from build123d import *

# Parameters (mm, degrees)
F1_DEPTH = 31.75
F2_DEPTH = 92.075
F0_R     = 15.875
F3_DEPTH = 53.975
F4_DEPTH = 73.025
F5_SCALE = 0.5


with BuildPart() as f1:
    # F0 (on Top) → F1 (new body)
    with BuildSketch(Plane.XY):
        Polygon((69.8498128911, -44.4499999985), (69.85, -76.2), (127, -76.2), (127, -25.4), (111.125, -25.4), (111.1241018772, 25.4), (126.9991018772, 25.4), (126.9991018772, 76.2), (69.8491018772, 76.2), (69.8492889861, 44.45), align=None)
    extrude(amount=F1_DEPTH)

    # F0 (on Top) → F2, piece 2 (join)
    with BuildSketch(Plane.XY):
        Polygon((38.1, 76.2), (38.1, 44.4498128953), (69.8492889861, 44.45), (69.8491018772, 76.2), align=None)
        Polygon((38.1, -44.4501871063), (38.1, -76.2), (69.85, -76.2), (69.8498128911, -44.4499999985), align=None)
    extrude(amount=F2_DEPTH)



with BuildPart() as f1b:
    # F0 (on Top) → F1, piece 2 (new body)
    with BuildSketch(Plane.XY):
        Polygon((-111.125, -25.4), (-127, -25.4), (-127, -76.2), (-69.85, -76.2), (-69.8501871089, -44.45), (-69.8507110139, 44.45), (-69.8508981228, 76.2), (-127.0008981228, 76.2), (-127.0008981228, 25.4), (-111.125, 25.4), align=None)
    extrude(amount=F1_DEPTH)

    # F0 (on Top) → F2 (join)
    with BuildSketch(Plane.XY):
        Polygon((-69.8508981228, 76.2), (-69.8507110139, 44.45), (-38.1, 44.45), (-38.1, 76.2), align=None)
        Polygon((-69.8501871089, -44.45), (-69.85, -76.2), (-38.1, -76.2), (-38.1, -44.45), align=None)
    extrude(amount=F2_DEPTH)


with BuildPart() as f1_1:
    add(f1.part)

    add(f1b.part)  # F3 merges F1b
    # F0 (on Top) → F3 (join)
    with BuildSketch(Plane.XY):
        Polygon((-38.1, -44.45), (-38.1, -76.2), (0, -76.2), (38.1, -76.2), (38.1, -44.4501871063), (38.1, 44.4498128953), (38.1, 76.2), (-38.1, 76.2), (-38.1, 44.45), align=None)
        Circle(F0_R, mode=Mode.SUBTRACT)
    extrude(amount=F3_DEPTH)

    # F0 (on Top) → F4 (join)
    with BuildSketch(Plane.XY):
        Polygon((38.1, 44.4498128953), (38.1, -44.4501871063), (69.8498128911, -44.4499999985), (69.8492889861, 44.45), align=None)
        Polygon((-69.8507110139, 44.45), (-69.8501871089, -44.45), (-38.1, -44.45), (-38.1, 44.45), align=None)
    extrude(amount=F4_DEPTH)


with BuildPart() as f1_2:
    # F5: moved
    add(f1_1.part.scale(F5_SCALE))


solid = f1_2.part
Design review of the part built by this model. Coordinates are the model's own, in mm. A direction names the side the tool comes from. Coordinates: 2 decimals unless noted, no trailing zeros. Order: outer loops, then holes, each group sorted by start corner. A loop starts at its lowest first (then second) coordinate and runs counter-clockwise, first axis right, second up.
Item 1: Take a section at A-A, the plane z = 29. Write out the cut boundary in (x, y) (3 decimals), then the cut area to 3 significant figures.
Item 2: For pin 1 Ø17.5 at (y, z) = (3.5, 10) entering from -X; pin 2 Ø24 at (y, z) = (-2, 33) entering from +X; pin 3 Ø5 at (x, y) = (24, -9) entering from +Z; pin 4 Ø14.5 at (x, y) = (0, 0) entering from -Z, all flat-tipped, find the tip position at first contact; note any pin that passes through.
Item 3: Take a section at C-C, the plane z = 41. Write out the cut boundary in (x, y) (3 decimals).
Item 4: For line 1 (Y direction, x = 0, z = 15.75); line 2 (X direction, y = 6, z = 30); line 3 (X direction, y = 24.5, z = 24), list the stretches that pass through material, from the lowest coordinate up.
Item 5: Take a section at B-B, the plane x = 0. Write out the cut boundary in (y, z).
Item 6: The part is to be moulded in two halves that separate along Y. For faces 1 (the flat face through (1, 38.1, 18)), 2 (the flat face through (19.05, 1, 34)), 3 (the flat face through (-27, 0, 36.512)), 4 (the flat face through (-1, -38.1, 18)), say which applies: pulls with the +Y half, pulls with the -Y half, needs draft (parallel to the pull), parting line crosses it, or undercut.
Item 7: For faces 5 (the flat face through (-49, 1, 15.875)), 6 (the flat face through (-55.562, 0, 8)), 7 (the flat face through (49, 1, 15.875)), 8 (the flat face through (8.2, 0.5, 26.988)), 9 (the flat face through (-27, 22.225, 41)), list the 3-axis set-ups (+Z, -Z, +X, -X, +Y, -Y) from which the entire face can be reached by the end or side of a thin tool; tool diameter is ignored.
The answers:
1. outline: (-34.925, -38.1) - (-19.05, -38.1) - (-19.05, 38.1) - (-34.925, 38.1) - close; (19.05, -38.1) - (34.925, -38.1) - (34.925, 38.1) - (19.05, 38.1) - close
1. area: 2,420 mm2
2. pin 1: stops at x = -55.56
2. pin 2: stops at x = 34.92
2. pin 3: stops at z = 36.51
2. pin 4: passes through
3. outline: (-34.925, -38.1) - (-19.05, -38.1) - (-19.05, -22.225) - (-34.925, -22.225) - close; (-34.925, 22.225) - (-19.05, 22.225) - (-19.05, 38.1) - (-34.925, 38.1) - close; (19.05, -38.1) - (34.925, -38.1) - (34.925, -22.225) - (19.05, -22.225) - close; (19.05, 22.225) - (34.925, 22.225) - (34.925, 38.1) - (19.05, 38.1) - close
4. line 1: y = -38.1 to -7.94, 7.94 to 38.1
4. line 2: x = -34.93 to -19.05, 19.05 to 34.92
4. line 3: x = -34.93 to 34.92
5. outline: (-38.1, 0) - (-7.94, 0) - (-7.94, 26.99) - (-38.1, 26.99) - close; (7.94, 0) - (38.1, 0) - (38.1, 26.99) - (7.94, 26.99) - close
6. face 1: pulls with the +Y half
6. face 2: needs draft
6. face 3: undercut
6. face 4: pulls with the -Y half
7. face 5: +Z, -X, +Y, -Y
7. face 6: +Z, -Z, -X
7. face 7: +Z, +X, +Y, -Y
7. face 8: +Z, +Y, -Y
7. face 9: +Z, +X, -X
